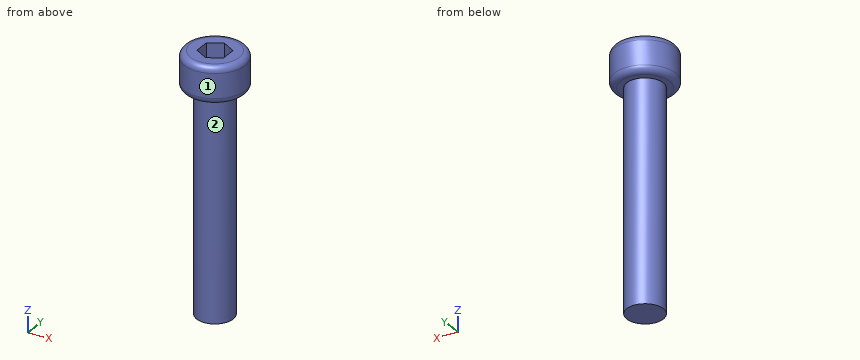
```python
from build123d import *

# Parameters (mm, degrees)
SKETCH1_R           = 1.5
BOSS_EXTRUDE1_DEPTH = 18
SKETCH2_R           = 2.5
BOSS_EXTRUDE2_DEPTH = 3
FILLET1_R           = 0.5
CUT_EXTRUDE1_DEPTH  = 2


with BuildPart() as part:
    # Sketch1 → Boss-Extrude1 (new body)
    with BuildSketch(Plane.XY):
        with Locations((0, 1.584180911)):
            Circle(SKETCH1_R)
    extrude(amount=-BOSS_EXTRUDE1_DEPTH)

    # Sketch2 → Boss-Extrude2 (add)
    with BuildSketch(Plane.XY):
        with Locations((0, 1.584180911)):
            Circle(SKETCH2_R)
    extrude(amount=BOSS_EXTRUDE2_DEPTH)

    # Fillet1
    fillet1_edges = [part.edges().sort_by_distance(p)[0] for p in [
        (-2.5, 1.584180911, 0),
        (-2.5, 1.584180911, 3),
    ]]
    fillet(fillet1_edges, radius=FILLET1_R)

    # Sketch3 → Cut-Extrude1 (cut)
    with BuildSketch(Plane.XY.offset(3)):
        Polygon((0, 0.320652174), (1.094247985, 0.952416543), (1.094247985, 2.21594528), (0, 2.847709649), (-1.094247985, 2.21594528), (-1.094247985, 0.952416543), align=None)
    extrude(amount=-CUT_EXTRUDE1_DEPTH, mode=Mode.SUBTRACT)


solid = part.part
```
For this review, take the finished solid that the model builds, in its own axes (mm). Face numbers are marked on the shaded views. A direction names the side the tool comes from. Coordinates: 2 decimals unless noted, no trailing zeros. Loops run counter-clockwise (first coordinate to the right, second up) from the corner with the lowest first, then second, coordinate; pieces in that order, holes last.
1. For line 1 (Z direction, x = 0.1, y = 3.45); line 2 (Y direction, x = -0.8, z = -16.5); line 3 (Z direction, x = 0.9, y = 1.1), list the stretches that pass through material, from the lowest coordinate up.
2. Add section B-B, the plane z = 0.75. Give the boundary of the cut face in (x, y), then the cut area to 3 significant figures.
3. For the marked faces 1 and 2, list the 3-axis set-ups (+Z, -Z, +X, -X, +Y, -Y) from which the entire face can be reached by the end or side of a thin tool; tool diameter is ignored.
4. Add section A-A, the plane z = -13.25. Give the boundary of the cut face in (x, y).
5. Insertion check: P1, Ø1.5, axis at x = 0, z = -9.5, coming from the +Y side; P2, Ø2, axis at y = 0.5, z = -8, coming from the +X side. Each pin has a flat end and moves straight along its axis. Give the tip position at first contact, or say it passes through.
Result:
1. line 1: z = 0 to 3
1. line 2: y = 0.32 to 2.85
1. line 3: z = -18 to 1
2. outline: circle Ø5 at (0, 1.58)
2. area: 19.6 mm2
3. face 1: +Z, -Z
3. face 2: -Z
4. outline: circle Ø3 at (0, 1.58)
5. P1: stops at y = 3.08
5. P2: stops at x = 1.5
